CAD build for the part. Positions are in the model's coordinates, mm. A direction names the side the tool comes from. Round coordinates to 2 decimals unless told otherwise and drop trailing zeros. Loops run counter-clockwise (first coordinate to the right, second up) from the corner with the lowest first, then second, coordinate; pieces in that order, holes last.
```python
from build123d import *

# Parameters (mm, degrees)
ESBO_O1_W                = 26
ESBO_O1_H                = 20
RESSALTO_EXTRUS_O1_DEPTH = 3
ESBO_O2_W                = 26
ESBO_O2_H                = 3
RESSALTO_EXTRUS_O2_DEPTH = 35
ESBO_O3_W                = 3
ESBO_O3_H                = 4.5
RESSALTO_EXTRUS_O3_DEPTH = 6
CORTE_EXTRUS_O1_DEPTH    = 48.329507785
CORTE_EXTRUS_O2_REACH    = 49.836
ESBO_O5_W                = 3.5
ESBO_O5_H                = 10
ESBO_O5_H_2              = 13
FILETE2_R                = 1.5
FILETE3_R                = 1.5
FILETE4_R                = 1.5
CORTE_EXTRUS_O3_REACH    = 46.815
ESBO_O6_W                = 7
ESBO_O6_H                = 3.5
FILETE5_R                = 1.5
CORTE_EXTRUS_O4_REACH    = 46.815
ESBO_O7_R                = 5.5


with BuildPart() as part:
    # Esbo_o1 → Ressalto-extrus_o1 (new body)
    with BuildSketch(Plane(origin=(0, 0, 0), x_dir=(1, 0, 0), z_dir=(0, 1, 0))):
        with Locations((8.077993659, -0.958207295)):
            Rectangle(ESBO_O1_W, ESBO_O1_H)
    extrude(amount=RESSALTO_EXTRUS_O1_DEPTH)

    # Esbo_o2 → Ressalto-extrus_o2 (add)
    with BuildSketch(Plane(origin=(0, 3, 0), x_dir=(1, 0, 0), z_dir=(0, 1, 0))):
        with Locations((8.077993659, -9.458207295)):
            Rectangle(ESBO_O2_W, ESBO_O2_H)
    extrude(amount=RESSALTO_EXTRUS_O2_DEPTH)

    # Esbo_o3 → Ressalto-extrus_o3 (add)
    with BuildSketch(Plane(origin=(0, 3, 0), x_dir=(1, 0, 0), z_dir=(0, 1, 0))):
        with Locations((19.577993659, -5.708207295)):
            Rectangle(ESBO_O3_W, ESBO_O3_H)
        with Locations((-3.422006341, -5.708207295)):
            Rectangle(ESBO_O3_W, ESBO_O3_H)
    extrude(amount=RESSALTO_EXTRUS_O3_DEPTH)

    # Esbo_o4 → Corte-extrus_o1 (cut, through all)
    with BuildSketch(Plane.ZY.offset(4.922006341)):
        Polygon((3.458207295, 3), (7.958207295, 9), (3.458207295, 9), align=None)
    extrude(amount=-CORTE_EXTRUS_O1_DEPTH, mode=Mode.SUBTRACT)

    # Esbo_o5 → Corte-extrus_o2 (cut, up to next)
    with BuildSketch(Plane.XY.offset(10.958207295), mode=Mode.PRIVATE) as corte_extrus_o2_sk1:
        with Locations((8.077993659, 29)):
            Rectangle(ESBO_O5_W, ESBO_O5_H)
    corte_extrus_o2_tool1 = extrude(corte_extrus_o2_sk1.sketch, amount=-CORTE_EXTRUS_O2_REACH, mode=Mode.PRIVATE) & part.part
    # Esbo_o5 → Corte-extrus_o2 (cut, up to next)
    with BuildSketch(Plane.XY.offset(10.958207295), mode=Mode.PRIVATE) as corte_extrus_o2_sk2:
        with Locations((8.077993659, 12.5)):
            Rectangle(ESBO_O5_W, ESBO_O5_H_2)
    corte_extrus_o2_tool2 = extrude(corte_extrus_o2_sk2.sketch, amount=-CORTE_EXTRUS_O2_REACH, mode=Mode.PRIVATE) & part.part
    add(corte_extrus_o2_tool1.solids().sort_by_distance((8.077994, 29, 10.958207))[0], mode=Mode.SUBTRACT)
    add(corte_extrus_o2_tool2.solids().sort_by_distance((8.077994, 12.5, 10.958207))[0], mode=Mode.SUBTRACT)

    # Filete2
    filete2_edges = [part.edges().sort_by_distance(p)[0] for p in [
        (6.327993659, 34, 9.458207295),
        (9.827993659, 34, 9.458207295),
        (9.827993659, 24, 9.458207295),
        (6.327993659, 24, 9.458207295),
        (6.327993659, 19, 9.458207295),
        (9.827993659, 19, 9.458207295),
    ]]
    fillet(filete2_edges, radius=FILETE2_R)

    # Filete3
    filete3_edges = [part.edges().sort_by_distance(p)[0] for p in [
        (6.327993659, 6, 9.458207295),
    ]]
    fillet(filete3_edges, radius=FILETE3_R)

    # Filete4
    filete4_edges = [part.edges().sort_by_distance(p)[0] for p in [
        (9.827993659, 6, 9.458207295),
    ]]
    fillet(filete4_edges, radius=FILETE4_R)

    # Esbo_o6 → Corte-extrus_o3 (cut, up to next)
    with BuildSketch(Plane.XZ, mode=Mode.PRIVATE) as corte_extrus_o3_sk1:
        with Locations((-4.922006341, 0.958207295)):
            Rectangle(ESBO_O6_W, ESBO_O6_H)
    corte_extrus_o3_tool1 = extrude(corte_extrus_o3_sk1.sketch, amount=-CORTE_EXTRUS_O3_REACH, mode=Mode.PRIVATE) & part.part
    # Esbo_o6 → Corte-extrus_o3 (cut, up to next)
    with BuildSketch(Plane.XZ, mode=Mode.PRIVATE) as corte_extrus_o3_sk2:
        with Locations((21.077993659, 0.958207295)):
            Rectangle(ESBO_O6_W, ESBO_O6_H)
    corte_extrus_o3_tool2 = extrude(corte_extrus_o3_sk2.sketch, amount=-CORTE_EXTRUS_O3_REACH, mode=Mode.PRIVATE) & part.part
    add(corte_extrus_o3_tool1.solids().sort_by_distance((-4.922006, 0, 0.958207))[0], mode=Mode.SUBTRACT)
    add(corte_extrus_o3_tool2.solids().sort_by_distance((21.077994, 0, 0.958207))[0], mode=Mode.SUBTRACT)

    # Filete5
    filete5_edges = [part.edges().sort_by_distance(p)[0] for p in [
        (-1.422006341, 1.5, 2.708207295),
        (-1.422006341, 1.5, -0.791792705),
        (17.577993659, 1.5, -0.791792705),
        (17.577993659, 1.5, 2.708207295),
    ]]
    fillet(filete5_edges, radius=FILETE5_R)

    # Esbo_o7 → Corte-extrus_o4 (cut, up to next)
    with BuildSketch(Plane.XZ, mode=Mode.PRIVATE) as corte_extrus_o4_sk1:
        with Locations(Location((8.077993659, 0.458207295, 0), (0, 0, 270))):
            Circle(ESBO_O7_R)
    corte_extrus_o4_tool1 = extrude(corte_extrus_o4_sk1.sketch, amount=-CORTE_EXTRUS_O4_REACH, mode=Mode.PRIVATE) & part.part
    add(corte_extrus_o4_tool1.solids().sort_by_distance((8.077994, 0, 0.458207))[0], mode=Mode.SUBTRACT)


solid = part.part
```
Item 1: Cut at B-B, the plane z = 8.5. Give the cut face in (x, y), plus the area to 3 significant figures.
Answers follow:
outline: (-4.92, 0) - (21.08, 0) - (21.08, 38) - (-4.92, 38) - close; hole (6.33, 7.5) arc R1.5 ccw to (7.83, 6) - (8.33, 6) arc R1.5 ccw to (9.83, 7.5) - (9.83, 17.5) arc R1.5 ccw to (8.33, 19) - (7.83, 19) arc R1.5 ccw to (6.33, 17.5) - close; hole (6.33, 25.5) arc R1.5 ccw to (7.83, 24) - (8.33, 24) arc R1.5 ccw to (9.83, 25.5) - (9.83, 32.5) arc R1.5 ccw to (8.33, 34) - (7.83, 34) arc R1.5 ccw to (6.33, 32.5) - close
area: 911 mm2
Item 2: Two-plate mould, pull along X, no slides. Class faces 6 (the flat face through (-1.922, 5, 6)), 7 (the flat face through (-4.922, 15, 9)), 8 (the flat face through (-4, 1, -0.792)): released by +X, released by -X, zero draft, split by the parting line, or undercut.
Answers follow:
face 6: undercut
face 7: released by -X
face 8: zero draft
Item 3: 3-axis set-ups, long thin cutter, end or side, ignore diameter. For faces 1 (the cylindrical face through (13.53, 1.48, 1.17)), 2 (the flat face through (20, 1, 2.708)), 3 (the flat face through (5, 3, -4.4)), 4 (the cylindrical face through (-1.87, 1.52, 2.28)), 5 (the cylindrical face through (6.756, 24.451, 9.437)): which of +Z, -Z, +X, -X, +Y, -Y reach the whole face in a straight line?
Answers follow:
face 1: +Y, -Y
face 2: +X, +Y, -Y
face 3: -Z, +Y
face 4: -X, +Y, -Y
face 5: +Z, -Z
Item 4: Cut at C-C, the plane z = 4.25. Give the cut face in (x, y), plus the area to 3 significant figures.
Answers follow:
outline: (-4.92, 0) - (4.09, 0) - (4.09, 3) - (-1.92, 3) - (-1.92, 4.06) - (-4.92, 4.06) - close; (12.06, 0) - (21.08, 0) - (21.08, 4.06) - (18.08, 4.06) - (18.08, 3) - (12.06, 3) - close
area: 60.4 mm2
Item 5: Flat gauge pins, fed straight in: P1, Ø4, axis at x = 14, y = 31.5, coming from the -Z side; P2, Ø3, axis at x = 7, z = -4, coming from the +Y side; P3, Ø1, axis at x = 10.5, z = -3, coming from the -Y side. Where does each tip first touch, or does it go through?
Answers follow:
P1: stops at z = 7.96
P2: stops at y = 3
P3: passes through
Item 6: Cut at A-A, the plane y = 17. Give the cut face in (x, z).
Answers follow:
outline: (-4.92, 7.96) - (6.33, 7.96) - (6.33, 10.96) - (-4.92, 10.96) - close; (9.83, 7.96) - (21.08, 7.96) - (21.08, 10.96) - (9.83, 10.96) - close
Item 7: Probe line 1 (X direction, y = 32.5, z = 9.5); line 2 (Y direction, x = 2.75, z = -2.25); line 3 (Z direction, x = 15, y = 21). List the from-to ranges inside material, lowest first.
Answers follow:
line 1: x = -4.92 to 6.33, 9.83 to 21.08
line 2: y = 0 to 3
line 3: z = 7.96 to 10.96
Item 8: Cut at D-D, the plane x = 14.75. Give the cut face in (y, z).
Answers follow:
outline: (0, -9.04) - (3, -9.04) - (3, 7.96) - (38, 7.96) - (38, 10.96) - (0, 10.96) - close
